from build123d import *

# Parameters (mm, degrees)
SKETCH2_W           = 30
SKETCH2_H           = 30
SKETCH2_R           = 1.75
BOSS_EXTRUDE1_DEPTH = 2
SKETCH3_W           = 30
SKETCH3_H           = 3
BOSS_EXTRUDE2_DEPTH = 76
SKETCH7_R           = 4
CUT_EXTRUDE1_DEPTH  = 3
SKETCH8_W           = 30
SKETCH8_H           = 2
CUT_EXTRUDE2_DEPTH  = 27
SKETCH9_W           = 3
SKETCH9_H           = 80
BOSS_EXTRUDE3_DEPTH = 33
SKETCH10_R          = 1.75
CUT_EXTRUDE3_DEPTH  = 37
CUT_EXTRUDE4_DEPTH  = 50
CUT_EXTRUDE5_REACH  = 38
SKETCH12_W          = 80
SKETCH12_H          = 10
SKETCH13_R          = 1.5
CUT_EXTRUDE6_DEPTH  = 6


with BuildPart() as part:
    # Sketch2 → Boss-Extrude1 (new body)
    with BuildSketch(Plane.XY):
        with Locations((-15, -15)):
            Rectangle(SKETCH2_W, SKETCH2_H)
        with Locations((-15, -2.5)):
            Circle(SKETCH2_R, mode=Mode.SUBTRACT)
    boss_extrude1 = extrude(amount=BOSS_EXTRUDE1_DEPTH)

    # Sketch3 → Boss-Extrude2 (add)
    with BuildSketch(Plane.XY.offset(2)):
        with Locations((-15, -28.5)):
            Rectangle(SKETCH3_W, SKETCH3_H)
    extrude(amount=BOSS_EXTRUDE2_DEPTH)

    # Mirror1: Boss-Extrude1 across plane
    add(boss_extrude1.mirror(Plane.XY.offset(40)))

    # Sketch7 → Cut-Extrude1 (cut)
    with BuildSketch(Plane(origin=(-25.653020371, -30, -8.772654641), x_dir=(1, 0, 0), z_dir=(0, -1, 0))):
        with Locations((10.653020371, 28.302654641)):
            Circle(SKETCH7_R)
    extrude(amount=-CUT_EXTRUDE1_DEPTH, mode=Mode.SUBTRACT)

    # Sketch8 → Cut-Extrude2 (cut)
    with BuildSketch(Plane(origin=(0, 0, 0), x_dir=(1, 0, 0), z_dir=(0, 1, 0))):
        with Locations((-15, -79)):
            Rectangle(SKETCH8_W, SKETCH8_H)
        with Locations((-15, -1)):
            Rectangle(SKETCH8_W, SKETCH8_H)
    extrude(amount=-CUT_EXTRUDE2_DEPTH, mode=Mode.SUBTRACT)

    # Sketch9 → Boss-Extrude3 (add)
    with BuildSketch(Plane.XZ.offset(30)):
        with Locations((1.5, 40)):
            Rectangle(SKETCH9_W, SKETCH9_H)
        with Locations((-31.5, 40)):
            Rectangle(SKETCH9_W, SKETCH9_H)
    extrude(amount=-BOSS_EXTRUDE3_DEPTH)

    # Sketch10 → Cut-Extrude3 (cut, through all)
    with BuildSketch(Plane.ZY.offset(33)):
        with Locations((40, 0)):
            Circle(SKETCH10_R)
    extrude(amount=-CUT_EXTRUDE3_DEPTH, mode=Mode.SUBTRACT)

    # Sketch11 → Cut-Extrude4 (cut)
    with BuildSketch(Plane(origin=(-33, -23.468882819, -8.772654641), x_dir=(0, 0, 1), z_dir=(-1, 0, 0))):
        with BuildLine():
            Line((47.095603657, 22.968882819), (46.522654641, 22.968882819))
            Line((46.522654641, 22.968882819), (46.522654641, 23.968882819))
            Line((46.522654641, 23.968882819), (47.095603657, 23.968882819))
            ThreePointArc((47.095603657, 23.968882819), (50.522654641, 23.468882819), (47.095603657, 22.968882819))
        make_face()
    extrude(amount=-CUT_EXTRUDE4_DEPTH, mode=Mode.SUBTRACT)

    # Sketch12 → Cut-Extrude5 (cut, up to next)
    with BuildSketch(Plane.ZY.offset(33), mode=Mode.PRIVATE) as cut_extrude5_sk1:
        with Locations((40, -2)):
            Rectangle(SKETCH12_W, SKETCH12_H)
    cut_extrude5_tool1 = extrude(cut_extrude5_sk1.sketch, amount=-CUT_EXTRUDE5_REACH, mode=Mode.PRIVATE) & part.part
    add(cut_extrude5_tool1.solids().sort_by_distance((-33, -2, 40))[0], mode=Mode.SUBTRACT)

    # Sketch13 → Cut-Extrude6 (cut)
    with BuildSketch(Plane(origin=(-36, -23.468882819, -8.772654641), x_dir=(0, 0, 1), z_dir=(-1, 0, 0))):
        with Locations((16.772654641, 11.468882819)):
            Circle(SKETCH13_R)
        with Locations((48.772654641, 11.468882819)):
            Circle(SKETCH13_R)
        with Locations((80.772654641, 11.468882819)):
            Circle(SKETCH13_R)
    extrude(amount=-CUT_EXTRUDE6_DEPTH, mode=Mode.SUBTRACT)


solid = part.part
Here's how the part is built. I have some questions about the finished solid (model axes, mm). A direction names the side the tool comes from. Coordinates: 2 decimals unless noted, no trailing zeros. Loops run counter-clockwise (first coordinate to the right, second up) from the corner with the lowest first, then second, coordinate; pieces in that order, holes last. Notation, with made-up numbers: (3.25, -12) -> (48.25, -12) arc R11 cw to (48.25, 7) -> close; hole circle Ø3 at (-34, 59.25). An arc over 180 degrees is marked (long way). Use one line per item in the form item = value. Start each with the question number.
(1) Please list where these lines run through material, in increasing order: line 1 along Y through (x, z) = (-31.5, 72); line 2 along X through (y, z) = (-26.5, 25); line 3 along Z through (x, y) = (-15, -29).
(2) If we section it at C-C (y = -19): Please give me the cut outline in (x, z), then the cut area to 3 significant figures.
(3) Will these pins go through, and if not, where does the flat tip stop? pin 1 (8 mm diameter, centred on x = -29, z = 65, fed in from +Y); pin 2 (1.5 mm diameter, centred on x = -26, z = 17, fed in from +Y); pin 3 (5 mm diameter, centred on y = -0.5, z = 52, fed in from -X); pin 4 (3 mm diameter, centred on y = 0, z = 40, fed in from +X).
(4) If we section it at D-D (x = -15): Please give me the cut outline in (y, z), then the cut area to 3 significant figures.
(5) On a 3-axis mill with a long thin cutter (end or side, diameter ignored), from which of +Z, -Z, +X, -X, +Y, -Y can I reach the whole of each face in a straight line? I mean faces 5 (the face through (-31.52, -11.55, 73.43)), 6 (the face through (-15, -27, 39)), 7 (the face through (1.48, -0.07, 41.75)). Say none if no direction works.
(6) If we section it at B-B (z = 40): Please give me the cut outline in (x, y), then the cut area to 4 significant figures.
(7) If we section it at A-A (y = -12): Please give me the cut outline in (x, z), then the cut area to 3 significant figures.
(8) We'd pull the mould along X, two halves only. Please class faces 1 (the face through (3, -14, 39)), 2 (the face through (-30, -17, 39)), 3 (the face through (-32, -7, 39)), 4 (the face through (-18.174, -28.521, 17.096)): pulls with the +X half, pulls with the -X half, needs draft (parallel to the pull), parting line crosses it, or undercut.
Verdict:
q1.line_1 = -30 to -13.5, -10.5 to -7
q1.line_2 = -33 to -30, 0 to 3
q1.line_3 = 0 to 15.53, 23.53 to 80
q2.outline = (-33, 0) -> (-30, 0) -> (-30, 80) -> (-33, 80) -> close; (0, 0) -> (3, 0) -> (3, 80) -> (0, 80) -> close
q2.area = 480 mm²
q3.pin_1 = -7
q3.pin_2 = -27
q3.pin_3 = 0
q3.pin_4 = through
q4.outline = (-30, 0) -> (-27, 0) -> (-27, 15.53) -> (-30, 15.53) -> close; (-30, 23.53) -> (-27, 23.53) -> (-27, 80) -> (-30, 80) -> close
q4.area = 216 mm²
q5.face_5 = -X
q5.face_6 = +Z, -Z, +Y
q5.face_7 = +X, -X
q6.outline = (-33, -30) -> (3, -30) -> (3, -1.75) -> (0, -1.75) -> (0, -27) -> (-30, -27) -> (-30, -13.5) -> (-33, -13.5) -> close; (-33, -10.5) -> (-30, -10.5) -> (-30, -7) -> (-33, -7) -> close; (0, 1.75) -> (3, 1.75) -> (3, 3) -> (0, 3) -> close
q6.area = 238.5 mm²
q7.outline = (-33, 0) -> (-30, 0) -> (-30, 6.5) -> (-33, 6.5) -> close; (-33, 9.5) -> (-30, 9.5) -> (-30, 38.5) -> (-33, 38.5) -> close; (-33, 41.5) -> (-30, 41.5) -> (-30, 70.5) -> (-33, 70.5) -> close; (-33, 73.5) -> (-30, 73.5) -> (-30, 80) -> (-33, 80) -> close; (0, 0) -> (3, 0) -> (3, 80) -> (0, 80) -> close
q7.area = 453 mm²
q8.face_1 = pulls with the +X half
q8.face_2 = undercut
q8.face_3 = needs draft
q8.face_4 = undercut
